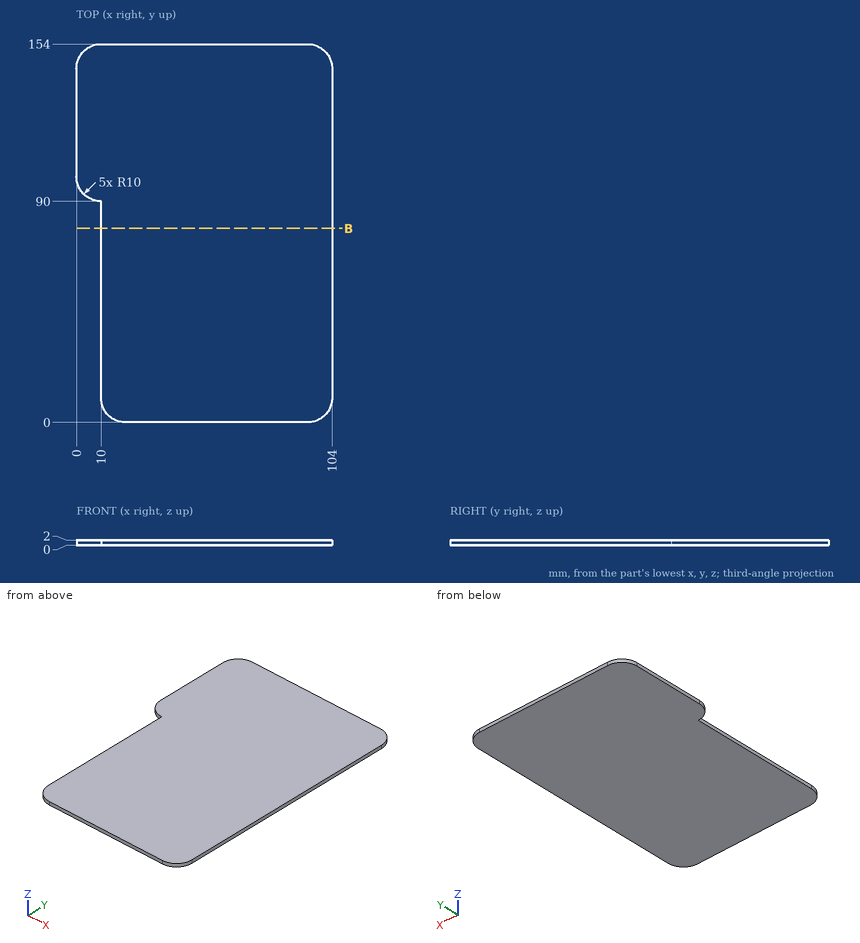
Could you check a few things on this drawing? It's one solid part, dimensions in mm from its lowest x, y, z. Round coordinates to 2 decimals unless told otherwise and drop trailing zeros. Order: outer loops, then holes, each group sorted by start corner. A loop starts at its lowest first (then second) coordinate and runs counter-clockwise, first axis right, second up. Notation, with made-up numbers: M 28.25,-36 L 79.25,-36 A18 ccw 79.25,-2 Z; hole C -30.75,39.5 d7. An arc over 180 degrees is marked long. Return JSON: item names as keys, results as strings. Group by question number.
1. I'm going to push a flat-ended pin straight in: pin 1 Ø8 at (x, y) = (67, 114.5) entering from -Z. Where does the tip first touch, or does it pass through?
2. If we section it at B-B on y = 79: List the corners of the cut face in (x, z) for me.
3. Please list where these lines run through material, in increasing order: probe 1 along X at (y, z) = (46.5, 1); probe 2 along Y at (x, z) = (14, 0.65); probe 3 along Y at (x, z) = (94.5, 0.1).
Reply:
{
 "1": {"pin 1": "z = 0"},
 "2": {"outline": "M 10,0 L 104,0 L 104,2 L 10,2 Z"},
 "3": {"probe 1": "10 to 104", "probe 2": "2 to 154", "probe 3": "0.01 to 153.99"}
}
